```python
from build123d import *

# Parameters (mm, degrees)
SKETCH1_R                = 20
SKETCH1_R_2              = 15
BOSS_EXTRUDE1_DEPTH      = 3
BOSS_EXTRUDE2_DEPTH      = 3
BOSS_EXTRUDE2_DEPTH_BACK = 3
BOSS_EXTRUDE3_DEPTH      = 3
BOSS_EXTRUDE3_DEPTH_BACK = 3
SKETCH4_R                = 1.25
BOSS_EXTRUDE4_DEPTH      = 3


with BuildPart() as part:
    # Sketch1 → Boss-Extrude1 (new body)
    with BuildSketch(Plane(origin=(0, 0, 0), x_dir=(1, 0, 0), z_dir=(0, 1, 0))):
        Circle(SKETCH1_R)
        Circle(SKETCH1_R_2, mode=Mode.SUBTRACT)
    extrude(amount=BOSS_EXTRUDE1_DEPTH)

    # Sketch2 → Boss-Extrude2 (add, two sides)
    with BuildSketch(Plane(origin=(0, 0, 0), x_dir=(0, 0, -1), z_dir=(1, 0, 0))) as boss_extrude2_sk:
        Polygon((20, 3), (17.979868871, 8), (7, 6.651841622), (7, 4.651841622), (15, 3), align=None)
        Polygon((-7, 4.651841622), (-15, 3), (-20, 3), (-17.979868871, 8), (-7, 6.651841622), align=None)
    extrude(amount=BOSS_EXTRUDE2_DEPTH)
    extrude(boss_extrude2_sk.sketch, amount=-BOSS_EXTRUDE2_DEPTH_BACK)

    # Sketch3 → Boss-Extrude3 (add, two sides)
    with BuildSketch(Plane.XY) as boss_extrude3_sk:
        Polygon((20, 3), (17.979868871, 8), (7, 6.651841622), (7, 4.651841622), (15, 3), align=None)
        Polygon((-7, 4.651841622), (-15, 3), (-20, 3), (-17.979868871, 8), (-7, 6.651841622), align=None)
    extrude(amount=BOSS_EXTRUDE3_DEPTH)
    extrude(boss_extrude3_sk.sketch, amount=-BOSS_EXTRUDE3_DEPTH_BACK)

    # Sketch4 → Boss-Extrude4 (add)
    with BuildSketch(Plane.XZ):
        with Locations((0, 18)):
            Circle(SKETCH4_R)
        with Locations((0, -18)):
            Circle(SKETCH4_R)
    extrude(amount=BOSS_EXTRUDE4_DEPTH)


solid = part.part
```
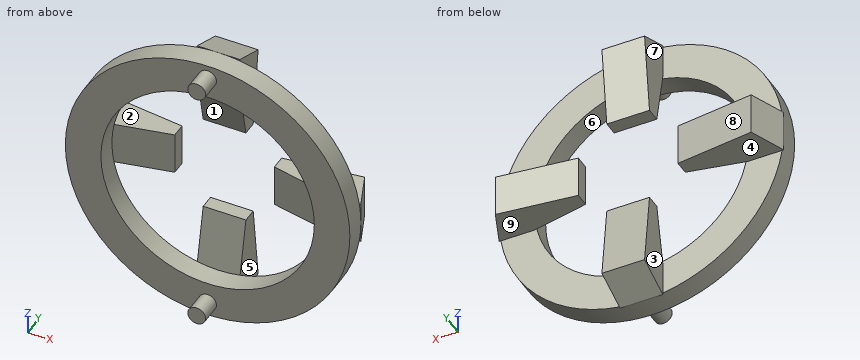
Input: part model. Units: mm. Frame: model coordinates. Face numbers are marked on the shaded views. A direction names the side the tool comes from. Give positions to 0.01 mm unless a question says otherwise; leave off trailing zeros. Loops run counter-clockwise (first coordinate to the right, second up) from the corner with the lowest first, then second, coordinate; pieces in that order, holes last. Notation, with made-up numbers: M -6,29.25 L 34,29.25 A15 cw 34,54.25 Z; hole C -20,-3.75 d11. An arc over 180 degrees is marked long. Answer as CSV lines item,"result". Start each with the question number.
1. Section D-D on y = -2.25. Return loops of the section in (x, z), plus the area to 3 significant figures.
2. Section B-B on z = -2.5. Return loops of the section in (x, y).
3. Line query: L1, parallel to Z at x = 0, y = 1.5; L2, parallel to Z at x = -18, y = 7. Output: solid intervals per line, ascending.
4. Section C-C on z = -12. Return loops of the section in (x, y), plus the area to 3 significant figures.
5. Pin query (flat end, axial travel): P1, Ø2.5, axis at x = 12, y = 6.5, coming from the -Z side; P2, Ø1.5, axis at y = 4.5, z = -16, coming from the -X side; P3, Ø5.5, axis at y = 4.5, z = 15.5, coming from the -X side. Return the tip coordinate at first contact, or that it passes through.
6. Pull-direction query (Z, two-part tool) for the marked faces 1, 2, 3 and 4; classes: released by +Z, released by -Z, zero draft, split by the parting line, or undercut.
7. Reachability of the marked faces 5, 6, 7, 8 and 9 from +Z, -Z, +X, -X, +Y, -Y: full face, straight path, thin tool, end or side. Return the list, or none.
8. Section A-A on x = -11. Return loops of the section in (y, z).
Computed values:
1,outline,"C 0,-18 d2.5; C 0,18 d2.5"
1,area,"9.82 mm²"
2,outline,"M -20,3 L -19.84,3 L -19.84,0 L -14.79,0 L -14.79,3 L -15,3 L -7,4.65 L -7,6.65 L -17.98,8 Z; M 7,4.65 L 15,3 L 14.79,3 L 14.79,0 L 19.84,0 L 19.84,3 L 20,3 L 17.98,8 L 7,6.65 Z"
3,L1,"z = -20 to -15, 15 to 20"
3,L2,"z = -3 to 3"
4,outline,"M -16,0 L -9,0 L -9,3 L -16,3 Z; M -3,3.62 L 3,3.62 L 3,7.27 L -3,7.27 Z; M 9,0 L 16,0 L 16,3 L 9,3 Z"
4,area,"63.9 mm²"
5,P1,"stops at z = -3"
5,P2,"stops at x = -3"
5,P3,"stops at x = -15.03"
6,face 1,"undercut"
6,face 2,"released by +Z"
6,face 3,"zero draft"
6,face 4,"released by -Z"
7,face 5,"+Z, -Z, +X, +Y"
7,face 6,"-Y"
7,face 7,"+Z, -Z, -X, +Y"
7,face 8,"+Z, -Z, +Y"
7,face 9,"-Z, +X, -X, +Y"
8,outline,"M 0,-16.7 L 3,-16.7 L 3,-10.2 L 0,-10.2 Z; M 0,10.2 L 3,10.2 L 3,16.7 L 0,16.7 Z; M 3.83,-3 L 7.14,-3 L 7.14,3 L 3.83,3 Z"
